The model under review builds one solid part; all positions refer to its coordinate system, in mm. Face numbers are marked on the shaded views. A direction names the side the tool comes from. Round coordinates to 2 decimals unless told otherwise and drop trailing zeros. Write each loop counter-clockwise with the first axis right and the second up, starting at its lowest first coordinate (ties: lowest second). Pieces come first, ordered by that corner, then holes. Notation, with made-up numbers: (74.25, -26) -> (107.25, -26) arc R14 cw to (107.25, -4) -> close; hole circle Ø2 at (40, -35.75). An arc over 180 degrees is marked (long way). Answer as a JSON object with one key per item and string values. Group by question number.
1) To check wall thickness, follow probe 1 along Z at (x, y) = (-4, -12); probe 2 along Z at (x, y) = (-24, -37.5); probe 3 along Y at (x, z) = (-90.5, 34). State the ranges of each line that lie inside material, in increasing order. Write a range as [from, to].
2) We need section B-B, the plane y = 0. Write out the cut boundary in (x, z), then the cut area to 3 significant figures.
3) We need section A-A, the plane x = 0. Write out the cut boundary in (y, z), then the cut area to 3 significant figures.
4) Mouldability with a two-part tool opening along X and no side actions: class the marked faces 1, 2 and 3 as pulls with the +X half, pulls with the -X half, needs draft (parallel to the pull), parting line crosses it, or undercut.
5) Machinability: for the marked faces 4, 5, 6, 7 and 8, which of the approach directions +Z, -Z, +X, -X, +Y, -Y give a long, thin tool a straight path to every point of the face, cutting with its end or side? Answer none if there is none.
6) We need section C-C, the plane z = 148. Write out the cut boundary in (x, y).
7) Insertion check: pin 1 Ø12 at (x, z) = (121, 136) entering from -Y; pin 2 Ø7.5 at (x, z) = (-126, 66) entering from -Y; pin 3 Ø9.5 at (y, z) = (5, 234) entering from -X. Each pin has a flat end and moves straight along its axis. Give the tip position at first contact, or say it passes through.
8) We need section D-D, the plane x = 120. Write out the cut boundary in (y, z), then the cut area to 3 significant figures.
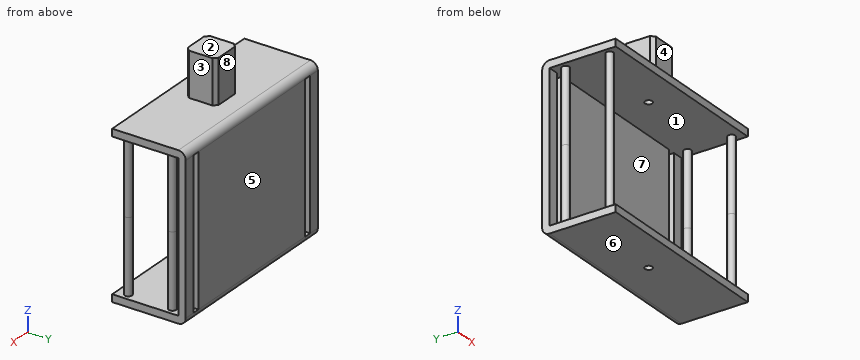
from build123d import *

# Parameters (mm, degrees)
SKETCH1_W                      = 130
SKETCH1_H                      = 45
SKETCH1_R                      = 5
BOSS_EXTRUDE1_DEPTH            = 10
SKETCH1_5_R                    = 5
BOSS_EXTRUDE2_DEPTH            = 100
MIRROR1_START                  = -10
MIRROR1_DEPTH                  = 10
MIRROR1_2_OUTLINE_R            = 5
MIRROR1_2_DEPTH                = 100
SKETCH2_W                      = 130
SKETCH2_H                      = 220
SKETCH2_W_2                    = 10
SKETCH2_H_2                    = 200
BOSS_EXTRUDE3_DEPTH            = 10
FILLET1_START                  = -131
FILLET1_DEPTH                  = 262
SKETCH3_W                      = 42
SKETCH3_H                      = 42
BOSS_EXTRUDE4_DEPTH            = 60
CHAMFER1_SIZE                  = 5
SKETCH4_R                      = 5
CUT_EXTRUDE1_DEPTH             = 10
CUT_EXTRUDE1_DIRECTION_2_REACH = 255.032


with BuildPart() as part:
    # Sketch1 → Boss-Extrude1 (new body)
    # profile 1 of 2: a face of its own
    with BuildSketch(Plane(origin=(0, 0, 0), x_dir=(1, 0, 0), z_dir=(0, 0, -1))):
        with Locations((-65, 22.5)):
            Rectangle(SKETCH1_W, SKETCH1_H)
        with Locations((-120, 30)):
            Circle(SKETCH1_R, mode=Mode.SUBTRACT)
    # profile 2 of 2: a face of its own
    with BuildSketch(Plane(origin=(0, 0, 0), x_dir=(1, 0, 0), z_dir=(0, 0, -1))):
        with Locations((-120, 30)):
            Circle(SKETCH1_R)
    extrude(amount=BOSS_EXTRUDE1_DEPTH)

    # Sketch1<5> → Boss-Extrude2 (add)
    with BuildSketch(Plane(origin=(0, 0, 0), x_dir=(1, 0, 0), z_dir=(0, 0, -1))):
        with Locations(Location((-120, 30, 0), (0, 0, 180))):
            Circle(SKETCH1_5_R)
    extrude(amount=-BOSS_EXTRUDE2_DEPTH)

    # Mirror1: read off the stored shape, not the designer's step
    # Mirror1 outline → Mirror1 (add)
    with BuildSketch(Plane.XY.offset(MIRROR1_START)):
        Polygon((130, 45), (-130, 45), (-130, 0), (0, 0), (0, -45), (130, -45), align=None)
    extrude(amount=MIRROR1_DEPTH)

    # Mirror1 2 outline → Mirror1 2 (add)
    with BuildSketch(Plane.XY):
        with Locations((120, -30)):
            Circle(MIRROR1_2_OUTLINE_R)
        with Locations((-120, 30)):
            Circle(MIRROR1_2_OUTLINE_R)
        with Locations((120, 30)):
            Circle(MIRROR1_2_OUTLINE_R)
    extrude(amount=MIRROR1_2_DEPTH)

    # Mirror2: part across plane


with BuildPart() as part_1:
    add(part.part)
    add(part.part.mirror(Plane(origin=(120, -30, 100), x_dir=(1, 0, 0), z_dir=(0, 0, -1))))

    # Sketch2 → Boss-Extrude3 (add)
    with BuildSketch(Plane(origin=(0, 45, 0), x_dir=(1, 0, 0), z_dir=(0, 1, 0))):
        with Locations((-65, -100)):
            Rectangle(SKETCH2_W, SKETCH2_H)
        with Locations((-110, -100)):
            Rectangle(SKETCH2_W_2, SKETCH2_H_2, mode=Mode.SUBTRACT)
    boss_extrude3 = extrude(amount=BOSS_EXTRUDE3_DEPTH)

    # Mirror3: Boss-Extrude3 across plane
    add(boss_extrude3.mirror(Plane(origin=(0, 55, -10), x_dir=(0, 0, 1), z_dir=(-1, 0, 0))))

    # Fillet1: read off the stored shape, not the designer's step
    # Fillet1 outline → Fillet1 (cut)
    with BuildSketch(Plane.YZ.offset(FILLET1_START)):
        with BuildLine():
            ThreePointArc((45, 210), (52.071067812, 207.071067812), (55, 200))
            Line((55, 200), (55, 210))
            Line((55, 210), (45, 210))
        make_face()
        with BuildLine():
            ThreePointArc((55, 0), (52.071067812, -7.071067812), (45, -10))
            Line((45, -10), (55, -10))
            Line((55, -10), (55, 0))
        make_face()
    extrude(amount=FILLET1_DEPTH, mode=Mode.SUBTRACT)

    # Sketch3 → Boss-Extrude4 (add)
    with BuildSketch(Plane.XY.offset(210)):
        Rectangle(SKETCH3_W, SKETCH3_H)
    extrude(amount=BOSS_EXTRUDE4_DEPTH)

    # Chamfer1
    chamfer1_edges = [part_1.edges().sort_by_distance(p)[0] for p in [
        (-21, -21, 240),
        (21, -21, 240),
        (21, 21, 240),
        (-21, 21, 240),
    ]]
    chamfer(chamfer1_edges, length=CHAMFER1_SIZE)

    # Sketch4 → Cut-Extrude1 (cut)
    with BuildSketch(Plane(origin=(0, 0, 200), x_dir=(-1, 0, 0), z_dir=(0, 0, -1))):
        with Locations(Location((0, 0, 0), (0, 0, 180))):
            Circle(SKETCH4_R)
    extrude(amount=-CUT_EXTRUDE1_DEPTH, mode=Mode.SUBTRACT)

    # Cut-Extrude1 direction 2: up to this face of the body (flat: up to its plane)
    cut_extrude1_direction_2_end = Plane(part_1.part.faces().sort_by_distance((0, 0, -10))[0])
    # Sketch4 → Cut-Extrude1 direction 2 (cut, up to the picked face)
    with BuildSketch(Plane(origin=(0, 0, 200), x_dir=(-1, 0, 0), z_dir=(0, 0, -1)), mode=Mode.PRIVATE) as cut_extrude1_direction_2_sk1:
        with Locations(Location((0, 0, 0), (0, 0, 180))):
            Circle(SKETCH4_R)
    cut_extrude1_direction_2_tool1 = split(extrude(cut_extrude1_direction_2_sk1.sketch, amount=CUT_EXTRUDE1_DIRECTION_2_REACH, mode=Mode.PRIVATE), bisect_by=cut_extrude1_direction_2_end, keep=Keep.BOTH, mode=Mode.PRIVATE)
    add(cut_extrude1_direction_2_tool1.solids().sort_by(Axis((0, 0, 200), (0, 0, -1)))[0], mode=Mode.SUBTRACT)


solid = part_1.part
Here are the results:
{
 "1": {"probe 1": "z = [-10, 0], [200, 270]", "probe 2": "z = [-10, 0], [200, 210]", "probe 3": "y = [45, 55]"},
 "2": {"outline": "(-130, -10) -> (-5, -10) -> (-5, 0) -> (-130, 0) -> close; (-130, 200) -> (-5, 200) -> (-5, 210) -> (5, 210) -> (5, 200) -> (130, 200) -> (130, 210) -> (21, 210) -> (21, 270) -> (-21, 270) -> (-21, 210) -> (-130, 210) -> close; (5, -10) -> (130, -10) -> (130, 0) -> (5, 0) -> close", "area": "7,520 mm^2"},
 "3": {"outline": "(-45, -10) -> (-5, -10) -> (-5, 0) -> (-45, 0) -> close; (-45, 200) -> (-5, 200) -> (-5, 210) -> (5, 210) -> (5, 200) -> (45, 200) -> (45, 0) -> (5, 0) -> (5, -10) -> (45, -10) arc R10 ccw to (55, 0) -> (55, 200) arc R10 ccw to (45, 210) -> (21, 210) -> (21, 270) -> (-21, 270) -> (-21, 210) -> (-45, 210) -> close", "area": "6,280 mm^2"},
 "4": {"face 1": "undercut", "face 2": "needs draft", "face 3": "pulls with the +X half"},
 "5": {"face 4": "+Z, +X, -X, -Y", "face 5": "+Z, -Z, +X, -X, +Y", "face 6": "-Z, +X, -X, +Y, -Y", "face 7": "+X, -X, -Y", "face 8": "+Z, +X, -X, +Y"},
 "6": {"outline": "(-130, 45) -> (-115, 45) -> (-115, 55) -> (-130, 55) -> close; circle Ø10 at (-120, -30); circle Ø10 at (-120, 30); (-105, 45) -> (105, 45) -> (105, 55) -> (-105, 55) -> close; circle Ø10 at (120, -30); circle Ø10 at (120, 30); (115, 45) -> (130, 45) -> (130, 55) -> (115, 55) -> close"},
 "7": {"pin 1": "stops at y = -35", "pin 2": "stops at y = -34.47", "pin 3": "stops at x = -21"},
 "8": {"outline": "(-45, -10) -> (45, -10) arc R10 ccw to (55, 0) -> (55, 200) arc R10 ccw to (45, 210) -> (-45, 210) -> (-45, 200) -> (-35, 200) -> (-35, 0) -> (-45, 0) -> close; hole (-25, 0) -> (25, 0) -> (25, 200) -> (-25, 200) -> close; hole (35, 0) -> (45, 0) -> (45, 200) -> (35, 200) -> close", "area": "7,960 mm^2"}
}
